from build123d import *

# Parameters (mm, degrees)
F0_W        = 23.7
F0_H        = 8
F0_R        = 2.5
F1_DEPTH    = 9.5
F2_DEPTH    = 2.2
F4_T        = -1.5
F5_R        = 3
F6_DEPTH    = 7.9248
F7_T        = 1
F7_T3_DEPTH = 10
F7_T5_DEPTH = 15
F7_T7_DEPTH = 22.7


# Not quite as in the source:
# - a shell that OpenCascade refuses in one call is made with other operations: the cavity is built on its own and cut out


with BuildPart() as f1:
    # F0 (on Top) → F1 (new body)
    with BuildSketch(Plane.XY):
        with Locations((11.85, 4)):
            Rectangle(F0_W, F0_H)
        with Locations((3.95, 4)):
            Circle(F0_R, mode=Mode.SUBTRACT)
        with Locations((11.85, 4)):
            Circle(F0_R, mode=Mode.SUBTRACT)
        with Locations((19.75, 4)):
            Circle(F0_R, mode=Mode.SUBTRACT)
        with Locations((19.75, 4)):
            Circle(F0_R)
        with Locations((11.85, 4)):
            Circle(F0_R)
        with Locations((3.95, 4)):
            Circle(F0_R)
    extrude(amount=-F1_DEPTH)

    # F0 (on Top) → F2 (join)
    with BuildSketch(Plane.XY):
        with Locations((3.95, 4)):
            Circle(F0_R)
        with Locations((11.85, 4)):
            Circle(F0_R)
        with Locations((19.75, 4)):
            Circle(F0_R)
    extrude(amount=F2_DEPTH)

    # F3: F1 across face


with BuildPart() as f1_1:
    add(f1.part)
    add(f1.part.mirror(Plane(origin=(11.85, 0, -4.75), x_dir=(1, 0, 0), z_dir=(0, -1, 0))))

    # F4
    f4_openings = [f1_1.faces().sort_by_distance(p)[0] for p in [
        (11.85, 0, -9.5),
    ]]
    offset(amount=F4_T, openings=f4_openings, kind=Kind.INTERSECTION)

    # F5 (on face) → F6 (join)
    with BuildSketch(Plane(origin=(0, 0, -1.5), x_dir=(1, 0, 0), z_dir=(0, 0, -1))):
        with Locations((8.3, 0)):
            Circle(F5_R)
        with Locations((15.4, 0)):
            Circle(F5_R)
    extrude(amount=F6_DEPTH)

    # F7: shell of thickness 1, made by hand


with BuildPart() as f7_core1:
    # F7_t2: copy of F1
    add(f1_1.part)

    # the walls: a layer under each face that stays
    f7_faces = [f7_core1.faces().sort_by_distance(p)[0] for p in [
        (0, 0, -4.75),
        (11.85, 8, -4.75),
        (1.6928571429, -6.8571428571, -9.5),
        (11.85, -8, -4.75),
        (11.85, 0, 0),
        (23.7, 0, -4.75),
        (1.5, 0, -5.5),
        (11.85, 6.5, -5.5),
        (22.2, 0, -5.5),
        (11.85, -6.5, -5.5),
        (1.45, 4, 1.1),
        (9.35, 4, 1.1),
        (17.25, 4, 1.1),
        (17.25, -4, 1.1),
        (1.45, -4, 1.1),
        (9.35, -4, 1.1),
        (11.85, 0, -1.5),
        (3.95, 4, 2.2),
        (11.85, 4, 2.2),
        (19.75, 4, 2.2),
        (19.75, -4, 2.2),
        (3.95, -4, 2.2),
        (11.85, -4, 2.2),
        (2.95, -4, -0.4),
        (10.85, -4, -0.4),
        (18.75, -4, -0.4),
        (5.3, 0, -5.4624),
        (2.95, 4, -0.4),
        (12.4, 0, -5.4624),
        (10.85, 4, -0.4),
        (18.75, 4, -0.4),
        (3.95, -4, 0.7),
        (11.85, -4, 0.7),
        (19.75, -4, 0.7),
        (3.95, 4, 0.7),
        (11.85, 4, 0.7),
        (19.75, 4, 0.7),
    ]]
    thicken(f7_faces, amount=-F7_T, mode=Mode.SUBTRACT)

    # F7_s4 → F7_t3 (cut)
    with BuildSketch(Plane.XY.offset(-10.5)):
        Polygon((1.51, 6.49), (0.5, 6.5), (0.5, 7.5), (1.5, 7.5), align=None)
        Polygon((1.51, -6.49), (0.5, -6.5), (0.5, -7.5), (1.5, -7.5), align=None)
        Polygon((22.19, 6.49), (22.2, 7.5), (23.2, 7.5), (23.2, 6.5), align=None)
        Polygon((22.19, -6.49), (23.2, -6.5), (23.2, -7.5), (22.2, -7.5), align=None)
    extrude(amount=F7_T3_DEPTH, mode=Mode.SUBTRACT)

    # F7_s6 → F7_t5 (cut)
    with BuildSketch(Plane.XZ.offset(-7.5)):
        Polygon((1.51, -1.51), (0.5, -1.5), (0.5, -0.5), (1.5, -0.5), align=None)
        Polygon((22.19, -1.51), (23.2, -1.5), (23.2, -0.5), (22.2, -0.5), align=None)
    extrude(amount=F7_T5_DEPTH, mode=Mode.SUBTRACT)

    # F7_s8 → F7_t7 (cut)
    with BuildSketch(Plane.YZ.offset(0.5)):
        Polygon((6.49, -1.51), (7.5, -1.5), (7.5, -0.5), (6.5, -0.5), align=None)
        Polygon((-6.49, -1.51), (-7.5, -1.5), (-7.5, -0.5), (-6.5, -0.5), align=None)
    extrude(amount=F7_T7_DEPTH, mode=Mode.SUBTRACT)

    # F7_s9 → F7_t10 (revolve, cut)
    with BuildSketch(Plane.XZ.offset(-4)):
        Polygon((6.46, 0.01), (6.45, -1), (5.45, -1), (5.45, 0), align=None)
    revolve(axis=Axis((3.95, 4, 0), (0, 0, 1)), mode=Mode.SUBTRACT)

    # F7_s11 → F7_t12 (revolve, cut)
    with BuildSketch(Plane.XZ.offset(-4)):
        Polygon((14.36, 0.01), (14.35, -1), (13.35, -1), (13.35, 0), align=None)
    revolve(axis=Axis((11.85, 4, 0), (0, 0, 1)), mode=Mode.SUBTRACT)

    # F7_s13 → F7_t14 (revolve, cut)
    with BuildSketch(Plane.XZ.offset(-4)):
        Polygon((22.26, 0.01), (22.25, -1), (21.25, -1), (21.25, 0), align=None)
    revolve(axis=Axis((19.75, 4, 0), (0, 0, 1)), mode=Mode.SUBTRACT)

    # F7_s15 → F7_t16 (revolve, cut)
    with BuildSketch(Plane.XZ.offset(4)):
        Polygon((22.26, 0.01), (22.25, -1), (21.25, -1), (21.25, 0), align=None)
    revolve(axis=Axis((19.75, -4, 0), (0, 0, -1)), mode=Mode.SUBTRACT)

    # F7_s17 → F7_t18 (revolve, cut)
    with BuildSketch(Plane.XZ.offset(4)):
        Polygon((6.46, 0.01), (6.45, -1), (5.45, -1), (5.45, 0), align=None)
    revolve(axis=Axis((3.95, -4, 0), (0, 0, -1)), mode=Mode.SUBTRACT)

    # F7_s19 → F7_t20 (revolve, cut)
    with BuildSketch(Plane.XZ.offset(4)):
        Polygon((14.36, 0.01), (14.35, -1), (13.35, -1), (13.35, 0), align=None)
    revolve(axis=Axis((11.85, -4, 0), (0, 0, -1)), mode=Mode.SUBTRACT)

    # F7_s21 → F7_t22 (revolve, cut)
    with BuildSketch(Plane.XZ):
        Polygon((11.31, -1.51), (11.3, -0.5), (10.3, -0.5), (10.3, -1.5), align=None)
    revolve(axis=Axis((8.3, 0, -1.5), (0, 0, -1)), mode=Mode.SUBTRACT)

    # F7_s23 → F7_t24 (revolve, cut)
    with BuildSketch(Plane.XZ):
        Polygon((18.41, -1.51), (18.4, -0.5), (17.4, -0.5), (17.4, -1.5), align=None)
    revolve(axis=Axis((15.4, 0, -1.5), (0, 0, -1)), mode=Mode.SUBTRACT)

    # F7_s25 → F7_t26 (revolve, cut)
    with BuildSketch(Plane.XZ.offset(4)):
        Polygon((4.94, 0.69), (5.95, 0.7), (5.95, 1.7), (4.95, 1.7), align=None)
    revolve(axis=Axis((3.95, -4, 0.7), (0, 0, -1)), mode=Mode.SUBTRACT)

    # F7_s27 → F7_t28 (revolve, cut)
    with BuildSketch(Plane.XZ.offset(4)):
        Polygon((12.84, 0.69), (13.85, 0.7), (13.85, 1.7), (12.85, 1.7), align=None)
    revolve(axis=Axis((11.85, -4, 0.7), (0, 0, -1)), mode=Mode.SUBTRACT)

    # F7_s29 → F7_t30 (revolve, cut)
    with BuildSketch(Plane.XZ.offset(4)):
        Polygon((20.74, 0.69), (21.75, 0.7), (21.75, 1.7), (20.75, 1.7), align=None)
    revolve(axis=Axis((19.75, -4, 0.7), (0, 0, -1)), mode=Mode.SUBTRACT)

    # F7_s31 → F7_t32 (revolve, cut)
    with BuildSketch(Plane.XZ.offset(-4)):
        Polygon((4.94, 0.69), (5.95, 0.7), (5.95, 1.7), (4.95, 1.7), align=None)
    revolve(axis=Axis((3.95, 4, 0.7), (0, 0, -1)), mode=Mode.SUBTRACT)

    # F7_s33 → F7_t34 (revolve, cut)
    with BuildSketch(Plane.XZ.offset(-4)):
        Polygon((12.84, 0.69), (13.85, 0.7), (13.85, 1.7), (12.85, 1.7), align=None)
    revolve(axis=Axis((11.85, 4, 0.7), (0, 0, -1)), mode=Mode.SUBTRACT)

    # F7_s35 → F7_t36 (revolve, cut)
    with BuildSketch(Plane.XZ.offset(-4)):
        Polygon((20.74, 0.69), (21.75, 0.7), (21.75, 1.7), (20.75, 1.7), align=None)
    revolve(axis=Axis((19.75, 4, 0.7), (0, 0, -1)), mode=Mode.SUBTRACT)


with BuildPart() as f1_2:
    add(f1_1.part)

    # what is left inside the walls is the cavity
    f7_cavity = [f7_core1.part.solids().sort_by_distance(p)[0] for p in [
        (13.41, 0, -3.808267),
        (6.31, 0, -3.808267),
    ]]
    add(f7_cavity, mode=Mode.SUBTRACT)


solid = f1_2.part
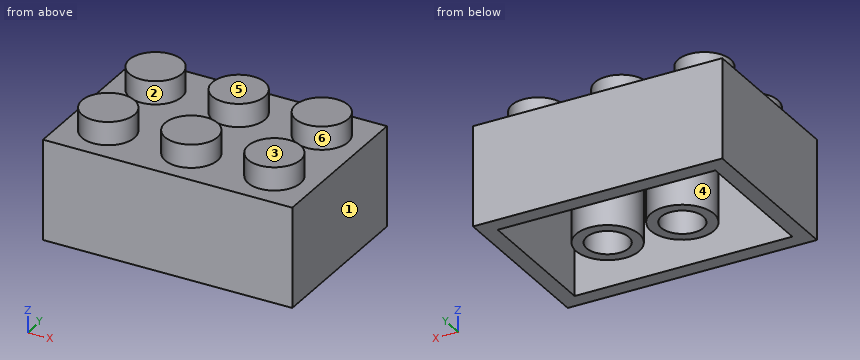
Geometry check sheet. Reference: the model listing, model coordinates, mm. Face numbers are marked on the shaded views. A direction names the side the tool comes from. Give positions to 0.01 mm unless a question says otherwise; leave off trailing zeros. Loops run counter-clockwise (first coordinate to the right, second up) from the corner with the lowest first, then second, coordinate; pieces in that order, holes last. Notation, with made-up numbers: M 59.5,48.25 L 72.5,48.25 A26 ccw 72.5,72.25 Z; hole C 21.5,-31 d4. An arc over 180 degrees is marked long. Answer as a JSON object with one key per item and string values. Group by question number.
Item 1: Gauge pin test, flat ends, axial feed: pin 1 (1.2 mm diameter, centred on x = 19.75, y = -4, fed in from -Z); pin 2 (1 mm diameter, centred on x = 17, y = 2, fed in from -Z); pin 3 (2 mm diameter, centred on x = 19.5, y = -3.5, fed in from -Z); pin 4 (5 mm diameter, centred on x = 3, y = 3, fed in from -Z). Record the tip position at first contact, or that the pin passes through.
Item 2: Sectioned sample at A-A on z = -1.75. Record the boundary of the cut face in (x, y), plus the area to 3 significant figures.
Item 3: Sectioned sample at B-B on z = -0.5. Record the boundary of the cut face in (x, y), plus the area to 3 significant figures.
Item 4: Sectioned sample at D-D on x = 8.3. Record the boundary of the cut face in (y, z), plus the area to 3 significant figures.
Item 5: Access from +Z, -Z, +X, -X, +Y, -Y to the whole of each face (thin tool, end or side, straight path). Record for the marked faces 4, 5 and 6.
Item 6: Mould release check, pull along X, two halves, no side actions. Record for the marked faces 1, 2 and 3: pulls with the +X half, pulls with the -X half, needs draft (parallel to the pull), parting line crosses it, or undercut.
Item 7: Material ranges on L1, parallel to Y at x = 19.75, z = 0.25; L2, parallel to Y at x = 19.75, z = -0.25; L3, parallel to X at y = 0, z = -7, recorded low to high.
Findings below:
{
 "1": {"pin 1": "z = 0.7", "pin 2": "z = -9.42", "pin 3": "z = -1.5", "pin 4": "z = -9.5"},
 "2": {"outline": "M 0,-8 L 23.7,-8 L 23.7,8 L 0,8 Z; C 8.3,0 d6; C 15.4,0 d6; hole M 1.5,-6.5 L 22.2,-6.5 L 22.2,6.5 L 1.5,6.5 Z; hole C 8.3,0 d4; hole C 15.4,0 d4", "area": "142 mm2"},
 "3": {"outline": "M 0,-8 L 23.7,-8 L 23.7,8 L 0,8 Z; hole C 3.95,-4 d2; hole C 3.95,4 d2; hole C 11.85,-4 d2; hole C 11.85,4 d2; hole C 19.75,-4 d2; hole C 19.75,4 d2", "area": "360 mm2"},
 "4": {"outline": "M -8,-9.5 L -6.5,-9.5 L -6.5,-1.5 L -3,-1.5 L -3,-9.42 L -2,-9.42 L -2,-1 L 2,-1 L 2,-9.42 L 3,-9.42 L 3,-1.5 L 6.5,-1.5 L 6.5,-9.5 L 8,-9.5 L 8,0 L -8,0 Z", "area": "61.8 mm2"},
 "5": {"face 4": "-Z", "face 5": "+Z, +X, -X, +Y, -Y", "face 6": "+Z"},
 "6": {"face 1": "pulls with the +X half", "face 2": "undercut", "face 3": "needs draft"},
 "7": {"L1": "-6.5 to -5, -3 to -1.5, 1.5 to 3, 5 to 6.5", "L2": "-8 to -5, -3 to 3, 5 to 8", "L3": "0 to 1.5, 5.3 to 6.3, 10.3 to 11.3, 12.4 to 13.4, 17.4 to 18.4, 22.2 to 23.7"}
}
